Input: dimensioned drawing with shaded views. Units: mm. Origin: part minimum x, y, z. Round coordinates to 2 decimals unless told otherwise and drop trailing zeros. Write each loop counter-clockwise with the first axis right and the second up, starting at its lowest first coordinate (ties: lowest second). Pieces come first, ordered by that corner, then holes. Notation, with made-up numbers: (38.5, 78) -> (79.5, 78) arc R30 ccw to (79.5, 108) -> close; hole circle Ø3 at (24, 76.25). An arc over 180 degrees is marked (long way). Use one line per item in the form item = value. Start each with the question number.
1. Cut plane D-D, the plane x = 104.5. Return the cut outline in (y, z).
2. Pin query (flat end, axial travel): pin 1 Ø1 at (x, z) = (21.5, 5) entering from +Y; pin 2 Ø2 at (y, z) = (160, 0.5) entering from +X; pin 3 Ø5.5 at (x, y) = (83.7, 170.1) entering from -Z (3 decimals); pin 4 Ø3 at (x, z) = (126, 3) entering from +Y. Return the tip coordinate at first contact, or that it passes through.
3. Cut plane A-A, the plane x = 51.3. Return the cut outline in (y, z).
4. Cut plane C-C, the plane x = 122.5. Return the cut outline in (y, z), plus the area to 3 significant figures.
5. Line query: L1, parallel to Y at x = 51.3, z = 4.35; L2, parallel to X at y = 146.95, z = 1.6 (3 decimals); L3, parallel to X at y = 170.1, z = 2.15. Output: solid intervals per line, ascending.
6. Cut plane B-B, the plane y = 170.1. Return the cut outline in (x, z).
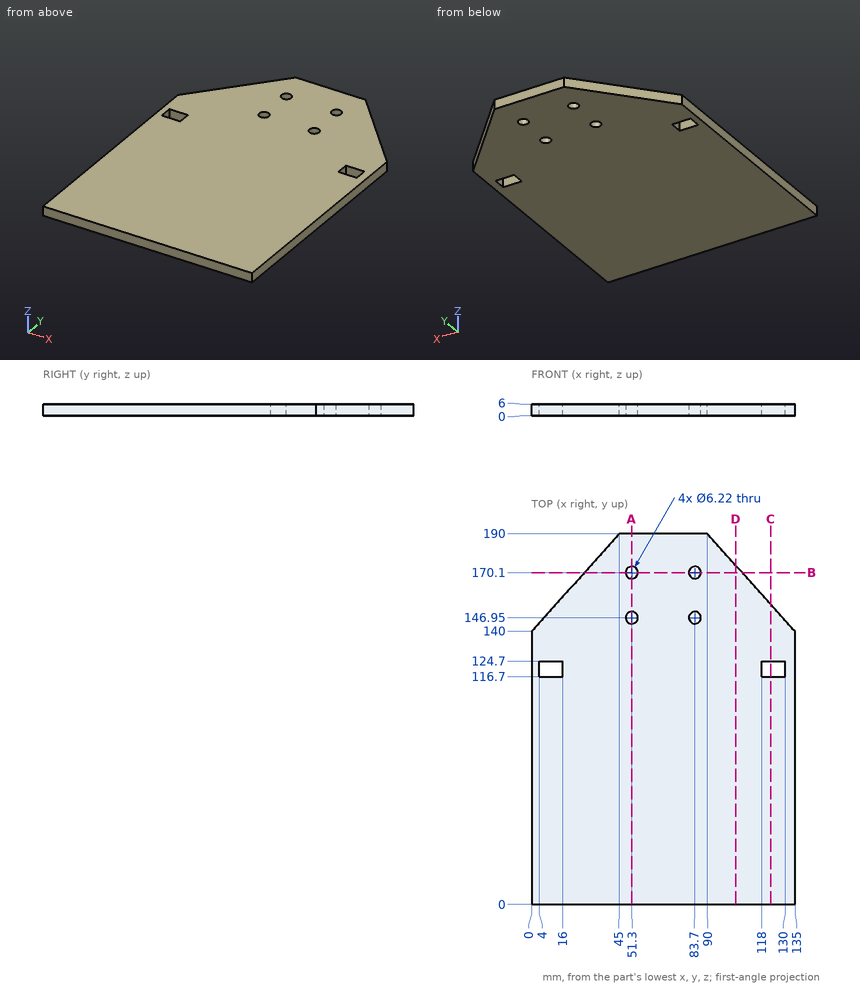
Outcome:
q1.outline = (0, 0) -> (173.89, 0) -> (173.89, 6) -> (0, 6) -> close
q2.pin_1 = 164.44
q2.pin_2 = 117.9
q2.pin_3 = through
q2.pin_4 = 151.67
q3.outline = (0, 0) -> (143.84, 0) -> (143.84, 6) -> (0, 6) -> close; (150.06, 0) -> (166.99, 0) -> (166.99, 6) -> (150.06, 6) -> close; (173.21, 0) -> (190, 0) -> (190, 6) -> (173.21, 6) -> close
q4.outline = (0, 0) -> (116.7, 0) -> (116.7, 6) -> (0, 6) -> close; (124.7, 0) -> (153.89, 0) -> (153.89, 6) -> (124.7, 6) -> close
q4.area = 875 mm^2
q5.L1 = 0 to 143.84, 150.06 to 166.99, 173.21 to 190
q5.L2 = 6.255 to 48.19, 54.41 to 80.59, 86.81 to 128.745
q5.L3 = 27.09 to 48.19, 54.41 to 80.59, 86.81 to 107.91
q6.outline = (27.09, 0) -> (48.19, 0) -> (48.19, 6) -> (27.09, 6) -> close; (54.41, 0) -> (80.59, 0) -> (80.59, 6) -> (54.41, 6) -> close; (86.81, 0) -> (107.91, 0) -> (107.91, 6) -> (86.81, 6) -> close
